Work out the finished part from the listing and answer in its coordinate system (mm). Round coordinates to 2 decimals unless told otherwise and drop trailing zeros. Order: outer loops, then holes, each group sorted by start corner. A loop starts at its lowest first (then second) coordinate and runs counter-clockwise, first axis right, second up. Notation, with made-up numbers: (-8, -29.5) - (43, -29.5) arc R15 ccw to (43, -16.5) - close; hole circle Ø3 at (83, 19.5). An arc over 180 degrees is marked (long way). Put each result on its own line as item: value.
```python
from build123d import *

# Parameters (mm, degrees)
SKETCH1_W           = 6.35
SKETCH1_H           = 25.4
BOSS_EXTRUDE1_DEPTH = 25.4
FILLET1_R           = 6.35
SKETCH2_R           = 11.1125
CUT_EXTRUDE1_DEPTH  = 7.35


with BuildPart() as part:
    # Sketch1 → Boss-Extrude1 (new body)
    with BuildSketch(Plane(origin=(0, 0, 0), x_dir=(1, 0, 0), z_dir=(0, 1, 0))):
        Rectangle(SKETCH1_W, SKETCH1_H)
    extrude(amount=BOSS_EXTRUDE1_DEPTH)

    # Fillet1
    fillet1_edges = [part.edges().sort_by_distance(p)[0] for p in [
        (0, 25.4, 12.7),
        (0, 25.4, -12.7),
    ]]
    fillet(fillet1_edges, radius=FILLET1_R)

    # Sketch2 → Cut-Extrude1 (cut, through all)
    with BuildSketch(Plane.ZY.offset(3.175)):
        with Locations((0, 13)):
            Circle(SKETCH2_R)
    extrude(amount=-CUT_EXTRUDE1_DEPTH, mode=Mode.SUBTRACT)


solid = part.part
```
1) A cutting plane is placed at C-C on y = 6. Write down the section's boundary in (x, z) (3 decimals).
Findings below:
outline: (-3.175, -12.7) - (3.175, -12.7) - (3.175, -8.631) - (-3.175, -8.631) - close; (-3.175, 8.631) - (3.175, 8.631) - (3.175, 12.7) - (-3.175, 12.7) - close
2) A cutting plane is placed at B-B on z = 0. Write down the section's boundary in (x, y) (1 decimal), then the cut area to 3 significant figures.
Findings below:
outline: (-3.2, 0) - (3.2, 0) - (3.2, 1.9) - (-3.2, 1.9) - close; (-3.2, 24.1) - (3.2, 24.1) - (3.2, 25.4) - (-3.2, 25.4) - close
area: 20.2 mm2
3) For a pull along Y with two mould halves and no side action, classify faces 1 (the cylindrical face through (-0.044, 24.018, -1.447)), 2 (the flat face through (0, 0, 0)), 3 (the cylindrical face through (0.04, 23.49, 10.89)), 4 (the flat face through (0, 9, 12.7)) as pulls with the +Y half, pulls with the -Y half, needs draft (parallel to the pull), parting line crosses it, or undercut.
Findings below:
face 1: undercut
face 2: pulls with the -Y half
face 3: pulls with the +Y half
face 4: needs draft
4) Straight lines are drawn through the part: L1, parallel to Y at x = -1.25, z = 0; L2, parallel to Y at x = 0.5, z = 7; L3, parallel to Z at x = 0, y = 17.75. For each, find the intervals that lie inside material, in ascending order. Write a range as from..to.
Findings below:
L1: y = 0..1.89, 24.11..25.4
L2: y = 0..4.37, 21.63..25.37
L3: z = -12.7..-10.05, 10.05..12.7
